Geometry: final body of the model. Coordinates: model frame, mm. A direction names the side the tool comes from. Coordinates: 2 decimals unless noted, no trailing zeros. Write each loop counter-clockwise with the first axis right and the second up, starting at its lowest first coordinate (ties: lowest second). Pieces come first, ordered by that corner, then holes.
Autodesk Inventor part; units mm, degrees
ref_plane "YZ Plane" through (0, 0, 0) normal (1, 0, 0) x (0, 1, 0)
ref_plane "XZ Plane" through (0, 0, 0) normal (0, 1, 0) x (-1, 0, 0)
ref_plane "XY Plane" through (0, 0, 0) normal (0, 0, 1) x (1, 0, 0)
sketch "Skizze1" plane through (0, 0, 0) normal (0, 1, 0) x (-1, 0, 0)
  line L0 (200, -150) -> (100, -150)
  line L1 (100, -150) -> (100, -30)
  line L2 (100, -30) -> (-100, -30)
  line L3 (-100, -30) -> (-100, -150)
  line L4 (-100, -150) -> (-200, -150)
  line L5 (-200, -150) -> (-200, -120)
  line L6 (-200, -120) -> (-130, -120)
  line L7 (-130, -120) -> (-130, 0)
  line L8 (-130, 0) -> (130, 0)
  line L9 (130, 0) -> (130, -120)
  line L10 (130, -120) -> (200, -120)
  line L11 (200, -120) -> (200, -150)
  line L12 (0, -180) -> (0, 30)
  point P0 (0, 0)
  dimension "d0" = 30
  dimension "d1" = 30
  dimension "d3" = 30
  dimension "d4" = 200
  dimension "d5" = 100
  dimension "d6" = 150
extrude "Extrusion1" add sketch "Skizze1" along normal blind 150
sketch "Skizze2" plane through (-130, 0, 0) normal (0, 0, 1) x (1, 0, 0)
  line L0 (230, 0) -> (30, 0)
  line L1 (55, 30) -> (205, 30)
  line L2 (205, 30) -> (205, 0)
  line L3 (205, 0) -> (55, 0)
  line L4 (55, 0) -> (55, 30)
  line L5 (260, 0) -> (260, 150)
  line L6 (0, 0) -> (0, 150)
  point P0 (130, 0)
  dimension "d9" = 260
  dimension "d10" = 30
  dimension "d11" = 150
  dimension "d12" = 55
extrude "Extrusion2" add sketch "Skizze2" along normal blind 300
sketch "Skizze3" plane through (0, 0, 0) normal (0, -1, 0) x (1, 0, 0)
  line L0 (-75, 300) -> (75, 300)
  line L1 (75, 0) -> (75, 300)
  line L2 (-75, 300) -> (75, 300)
  line L3 (75, 300) -> (75, 270)
  line L4 (75, 270) -> (-75, 270)
  line L5 (-75, 270) -> (-75, 300)
  point P0 (0, 0)
  dimension "d15" = 30
extrude "Extrusion3" add sketch "Skizze3" along normal blind 400
sketch "Skizze4" plane through (-130, 0, 300) normal (0, 0, 1) x (1, 0, 0)
  line L0 (110, -355) -> (150, -355)
  line L1 (150, -355) -> (150, -335)
  line L2 (150, -335) -> (110, -335)
  line L3 (110, -335) -> (110, -355)
  line L4 (110, -355) -> (150, -335) construction
  line L5 (150, -355) -> (110, -335) construction
  point P0 (130, 0)
  point P1 (130, -345)
  dimension "d18" = 40
  dimension "d19" = 20
  dimension "d20" = 345
  dimension "d21" = 0
extrude "Extrusion4" cut sketch "Skizze4" against normal through all
equation "\"d1\" = d0"
equation "\"d3\" = d0"
equation "\"d12\" = -0.5 * d11 + 0.5 * d9"
properties part number "Staender"
Item 1: Section A-A, the plane z = -82.5. Output: boundary loops of the cut face in (x, y).
Derived:
outline: (-130, 0) - (-100, 0) - (-100, 150) - (-130, 150) - close; (100, 0) - (130, 0) - (130, 150) - (100, 150) - close
Item 2: Pull-direction query (Y, two-part tool) for faces 1 (the flat face through (20, -345, 285)), 2 (the flat face through (0, -355, 285)), 3 (the flat face through (-14, 0, 61)), 4 (the flat face through (1, -197, 270)); classes: released by +Y, released by -Y, zero draft, split by the parting line, or undercut.
Derived:
face 1: undercut
face 2: undercut
face 3: released by -Y
face 4: zero draft
Item 3: Material intervals for probe 1 along X at (y, z) = (69, -126); probe 2 along Y at (x, z) = (62, 23.5); probe 3 along Y at (x, z) = (10, -8), sorted ascending.
Derived:
probe 1: x = -200 to -100, 100 to 200
probe 2: y = 0 to 30
probe 3: y = 0 to 150
Item 4: Section D-D, the plane z = 170.5. Output: boundary loops of the cut face in (x, y).
Derived:
outline: (-75, 0) - (75, 0) - (75, 30) - (-75, 30) - close
Item 5: Set-up query: faces 5 (the flat face through (165, 74, -120)), 6 (the flat face through (-1, 74, -30)), 7 (the flat face through (0, -335, 285)). Return all of +Z, -Z, +X, -X, +Y, -Y with unobstructed straight access to the full face (end or side cutting, diameter ignored); none if empty.
Derived:
face 5: +Z, +X, +Y, -Y
face 6: -Z, +Y, -Y
face 7: +Z, -Z
Item 6: Pin query (flat end, axial travel): pin 1 (3 mm diameter, centred on x = -14, y = -273.5, fed in from -Z); pin 2 (21 mm diameter, centred on x = -179, y = 70.5, fed in from +Z); pin 3 (8 mm diameter, centred on y = 14, z = -15.5, fed in from +X). Return the tip coordinate at first contact, or that it passes through.
Derived:
pin 1: stops at z = 270
pin 2: stops at z = -120
pin 3: stops at x = 130
Item 7: Section C-C, the plane y = -314. Output: boundary loops of the cut face in (x, z), plus the area to 3 significant figures.
Derived:
outline: (-75, 270) - (75, 270) - (75, 300) - (-75, 300) - close
area: 4,500 mm2
Item 8: Section B-B, the plane x = -38. Output: boundary loops of the cut face in (y, z).
Derived:
outline: (-400, 270) - (0, 270) - (0, -30) - (150, -30) - (150, 0) - (30, 0) - (30, 300) - (-400, 300) - close
